from build123d import *

# Parameters (mm, degrees)
BOSS_EXTRUDE1_DEPTH         = 7.62
CUT_EXTRUDE1_START          = 1.523953
CUT_EXTRUDE1_DEPTH          = 0.508
F_1_4_0_25_DIAMETER_HOLE1_D = 6.35
CHAMFER1_SIZE               = 0.254


# Read off the part's stored shape, not the designer's step: CSK for #6 Flat Head Machine Screw (100)1, CSK for #6 Flat Head Machine Screw (100)2
with BuildPart() as part:
    # Sketch1 → Boss-Extrude1 (new body)
    with BuildSketch(Plane(origin=(0, 0, 0), x_dir=(-1, 0, 0), z_dir=(0, 0, -1))):
        with BuildLine():
            Line((10.16, -6.506813736), (10.16, 6.506813736))
            ThreePointArc((10.16, 6.506813736), (8.531243315, 8.531243315), (6.506813736, 10.16))
            Line((6.506813736, 10.16), (-6.506813736, 10.16))
            ThreePointArc((-6.506813736, 10.16), (-8.531243315, 8.531243315), (-10.16, 6.506813736))
            Line((-10.16, 6.506813736), (-10.16, -6.506813736))
            ThreePointArc((-10.16, -6.506813736), (-8.531243315, -8.531243315), (-6.506813736, -10.16))
            Line((-6.506813736, -10.16), (6.506813736, -10.16))
            ThreePointArc((6.506813736, -10.16), (8.531243315, -8.531243315), (10.16, -6.506813736))
        make_face()
    extrude(amount=-BOSS_EXTRUDE1_DEPTH)

    # Sketch2 → Cut-Extrude1 (cut)
    with BuildSketch(Plane(origin=(0, 0, 1.523952559), x_dir=(-1, 0, 0), z_dir=(0, 0, -1)).offset(CUT_EXTRUDE1_START)):
        with BuildLine():
            Line((1.889125, -8.001), (1.158875, -8.001))
            add(Edge.make_bspline(
                [(1.158875, -8.001), (1.158872937, -8.044475215), (1.158868812, -8.131425646), (1.158899751, -8.261853836), (1.158782182, -8.392271851), (1.159221519, -8.522728024), (1.157581766, -8.65303983), (1.163686315, -8.783563395), (1.131096282, -8.911728677), (1.058473502, -9.021898611), (0.953640515, -9.101760404), (0.829437405, -9.145385371), (0.697588706, -9.145896155), (0.573131645, -9.103398602), (0.467813448, -9.024298708), (0.394265073, -8.914779016), (0.360421234, -8.786730663), (0.366393811, -8.655863654), (0.36478471, -8.525077993), (0.365216149, -8.394030645), (0.365100694, -8.26302727), (0.365131077, -8.132012169), (0.365127026, -8.044670723), (0.365125, -8.001)],
                knots=[0, 0, 0, 0, 0.04771921, 0.095438419, 0.143157629, 0.190876839, 0.238596048, 0.286313163, 0.333682366, 0.381043764, 0.428414282, 0.475836339, 0.523086151, 0.570387621, 0.617736793, 0.665150189, 0.712504193, 0.760330872, 0.808264698, 0.856198523, 0.904132349, 0.952066174, 1, 1, 1, 1], degree=3))
            Line((0.365125, -8.001), (-1.889125, -8.001))
            add(Edge.make_bspline(
                [(-1.889125, -8.001), (-1.889114812, -8.051894525), (-1.889094436, -8.153683576), (-1.889247255, -8.306368158), (-1.888666545, -8.459048717), (-1.890836563, -8.611744064), (-1.882759373, -8.763965749), (-1.914911349, -8.916005254), (-2.006583536, -9.041712954), (-2.136758982, -9.125851008), (-2.289345509, -9.153077401), (-2.441459117, -9.123368959), (-2.569808734, -9.037082272), (-2.65983821, -8.910286231), (-2.688880942, -8.757615863), (-2.681256155, -8.60511048), (-2.683310175, -8.451698443), (-2.682753256, -8.298343213), (-2.682926802, -8.144961863), (-2.682789537, -7.991619884), (-2.683165051, -7.838146541), (-2.681801975, -7.685351504), (-2.686853196, -7.53117355), (-2.628890851, -7.38497772), (-2.521046133, -7.273065177), (-2.378348767, -7.206351642), (-2.223808502, -7.207490017), (-2.072112792, -7.207185716), (-1.919779713, -7.207267225), (-1.767631713, -7.207245385), (-1.615434122, -7.207251236), (-1.463249814, -7.20724967), (-1.311061964, -7.207250082), (-1.209603988, -7.207250027), (-1.158875, -7.20725)],
                knots=[0, 0, 0, 0, 0.031320452, 0.062640904, 0.093961356, 0.125281809, 0.156602077, 0.187665627, 0.218747437, 0.249771849, 0.28082955, 0.311809013, 0.342800401, 0.373834649, 0.404881688, 0.436337896, 0.467799211, 0.499260526, 0.530721841, 0.562183156, 0.593644471, 0.625105786, 0.656448512, 0.68765108, 0.718839254, 0.750218434, 0.781469964, 0.81268854, 0.843907117, 0.875125693, 0.90634427, 0.937562847, 0.968781423, 1, 1, 1, 1], degree=3))
            add(Edge.make_bspline(
                [(-1.158875, -7.20725), (-1.158873643, -7.162894388), (-1.158870928, -7.074183165), (-1.158891289, -6.941111847), (-1.158813917, -6.808058432), (-1.159103046, -6.674937496), (-1.158160413, -6.542105789), (-1.162792352, -6.40859388), (-1.123081204, -6.279296809), (-1.043328982, -6.17099473), (-0.932633409, -6.094593309), (-0.802795792, -6.059099197), (-0.668632801, -6.067681678), (-0.544609192, -6.120335348), (-0.445331921, -6.210309856), (-0.378114798, -6.328380261), (-0.369456887, -6.416856776), (-0.365125, -6.461125)],
                knots=[0, 0, 0, 0, 0.066968294, 0.133936588, 0.200904882, 0.267873219, 0.334841936, 0.401752492, 0.468337617, 0.534646563, 0.601246412, 0.66759139, 0.734141278, 0.800523112, 0.867014877, 0.933462398, 1, 1, 1, 1], degree=3))
            Line((-0.365125, -6.461125), (-0.365125, -7.20725))
            add(Edge.make_bspline(
                [(-0.365125, -7.20725), (-0.31073924, -7.20725), (-0.20196772, -7.20725), (-0.03881044, -7.20725), (0.124346841, -7.20725), (0.287504121, -7.20725), (0.450661401, -7.207250001), (0.61381868, -7.207249996), (0.776975966, -7.207250014), (0.940133226, -7.207249949), (1.103290581, -7.207250189), (1.26644758, -7.207249293), (1.42960591, -7.207252638), (1.59275927, -7.207240153), (1.755931181, -7.207286749), (1.91903386, -7.207112852), (2.082398735, -7.207761857), (2.244713636, -7.205340907), (2.410623595, -7.213297949), (2.556377817, -7.298886101), (2.658013084, -7.432947287), (2.689729238, -7.59799594), (2.681031241, -7.762226985), (2.683361321, -7.927506447), (2.682773435, -8.092675694), (2.682794937, -8.257881374), (2.683296815, -8.423048668), (2.68126756, -8.588352833), (2.688866329, -8.75283629), (2.658381139, -8.918643331), (2.555396264, -9.053764707), (2.408701771, -9.136770112), (2.2405432, -9.153020414), (2.080098519, -9.09990658), (1.955237034, -8.986695), (1.885247755, -8.831155243), (1.890172169, -8.664016711), (1.888843871, -8.498928973), (1.889199968, -8.332843432), (1.889106258, -8.166945119), (1.889118753, -8.05631504), (1.889125, -8.001)],
                knots=[0, 0, 0, 0, 0.025504461, 0.051008922, 0.076513383, 0.102017844, 0.127522304, 0.153026765, 0.178531226, 0.204035687, 0.229540148, 0.255044609, 0.28054907, 0.306053531, 0.331557991, 0.357062452, 0.382566913, 0.408073163, 0.433537274, 0.459042456, 0.484570707, 0.510085466, 0.535909525, 0.561732239, 0.587554953, 0.613377667, 0.639200381, 0.665023095, 0.690855069, 0.716494274, 0.742192433, 0.767783402, 0.793488921, 0.819098849, 0.844763736, 0.870443974, 0.896243874, 0.922182905, 0.948121937, 0.974060968, 1, 1, 1, 1], degree=3))
        make_face()
    extrude(amount=-CUT_EXTRUDE1_DEPTH, mode=Mode.SUBTRACT)

    # Sketch3 → Revolve1 (revolve)
    with BuildSketch(Plane.XZ, mode=Mode.PRIVATE) as revolve1_sk:
        Polygon((9.4615, 20.32), (0, 20.32), (0, 7.62), (9.525, 7.62), (9.525, 17.78), (8.9408, 17.78), (8.9408, 19.05), (9.4615, 19.05), align=None)
    revolve(revolve1_sk.sketch.rotate(Axis((0, 0, 20.32), (0, 0, -1)), 180), axis=Axis((0, 0, 20.32), (0, 0, -1)))

    # 1/4 (0.25) Diameter Hole1 (through all)
    with Locations(Plane(origin=(0, 0, 0), x_dir=(-1, 0, 0), z_dir=(0, 0, -1))):
        with Locations((0, 0)):
            Hole(F_1_4_0_25_DIAMETER_HOLE1_D / 2)

    # CSK for _6 Flat Head Machine Screw _ 2 → CSK for _6 Flat Head Machine Screw _100 (revolve, cut)
    with BuildSketch(Plane(origin=(0, 0, 3.81), x_dir=(0.7071067811866009, 0.7071067811864942, 0), z_dir=(0, 0, -1))):
        Polygon((2.0828, -8.509), (2.0828, -2.395972613), (0, -2.395972613), (0, -12.065031051), (2.2479, -12.065031051), (2.2479, -8.577386659), align=None)
    revolve(axis=Axis((0, 0, 3.81), (0.7071067811864942, -0.7071067811866009, 0)), mode=Mode.SUBTRACT)

    # CSK for _6 Flat Head Machine Screw _ 3 o → CSK for _6 Flat Head Machine Screw _ 3 (revolve, cut)
    with BuildSketch(Plane(origin=(0, 0, 3.81), x_dir=(0.707106781186431, -0.707106781186664, 0), z_dir=(0, 0, 1))):
        Polygon((0, 2.395972613), (2.0828, 2.395972613), (2.0828, 8.509), (2.2479, 8.577386659), (2.2479, 12.065031051), (0, 12.065031051), align=None)
    revolve(axis=Axis((0, 0, 3.81), (0.707106781186664, 0.707106781186431, 0)), mode=Mode.SUBTRACT)

    # Chamfer1
    chamfer1_edges = [part.edges().sort_by_distance(p)[0] for p in [
        (9.4615, 0, 20.32),
        (-3.175, 0, 0),
        (-3.175, 0, 20.32),
    ]]
    chamfer(chamfer1_edges, length=CHAMFER1_SIZE)


solid = part.part
Source: CAD feature listing. Evaluate the final solid. Frame: model axes, mm. A direction names the side the tool comes from. Round coordinates to 2 decimals unless told otherwise and drop trailing zeros. Loops run counter-clockwise (first coordinate to the right, second up) from the corner with the lowest first, then second, coordinate; pieces in that order, holes last.
Q1. First-contact query: P1, Ø2, axis at x = -0.5, y = -0.5, coming from the +Z side; P2, Ø5, axis at y = -7.5, z = 12.5, coming from the +X side; P3, Ø0.6, axis at y = -7, z = 0.5, coming from the +X side. Flat tips, straight axial feed; report the tip coordinate or a pass-through.
Q2. Access query for faces 4 (the face through (1.938, -8.728, 18.424)), 5 (the face through (0, 5, 0)). Directions: +Z, -Z, +X, -X, +Y, -Y. A direction counts if a zero-diameter tool reaches every point of the face in a straight line with its end or side. Return the directions, or none.
Q3. Mould query, pull axis Y, two halves, no side actions, for faces 1 (the face through (2.06, -9.3, 12.77)), 2 (the face through (3.567, 4.205, 5.843)), 3 (the face through (-7.249, 9.644, 2.063)). Classes: pulls with the +Y half, pulls with the -Y half, needs draft (parallel to the pull), parting line crosses it, or undercut.
Q4. Section B-B, the plane z = 11.5. Return loops of the section in (x, y) (3 decimals).
Q5. Section A-A, the plane z = 18.5. Return loops of the section in (x, y) (3 decimals).
Q6. Ray query, line 1 (Y direction, x = 0, z = 13.5) (3 decimals); line 2 (Z direction, x = -2, y = -8.75); line 3 (Y direction, x = 0, z = 6.5) (3 decimals). Return the intervals inside material, ascending.
Solutions:
1. P1: passes through
1. P2: stops at x = 8.11
1. P3: stops at x = 10.03
2. face 4: none
2. face 5: -Z, +X, -X, +Y, -Y
3. face 1: parting line crosses it
3. face 2: undercut
3. face 3: pulls with the +Y half
4. outline: circle Ø19.05 at (0, 0); hole circle Ø6.35 at (0, 0)
5. outline: circle Ø17.882 at (0, 0); hole circle Ø6.35 at (0, 0)
6. line 1: y = -9.525 to -3.175, 3.175 to 9.525
6. line 2: z = 0.51 to 17.78, 19.05 to 20.32
6. line 3: y = -10.16 to -3.175, 3.175 to 10.16
